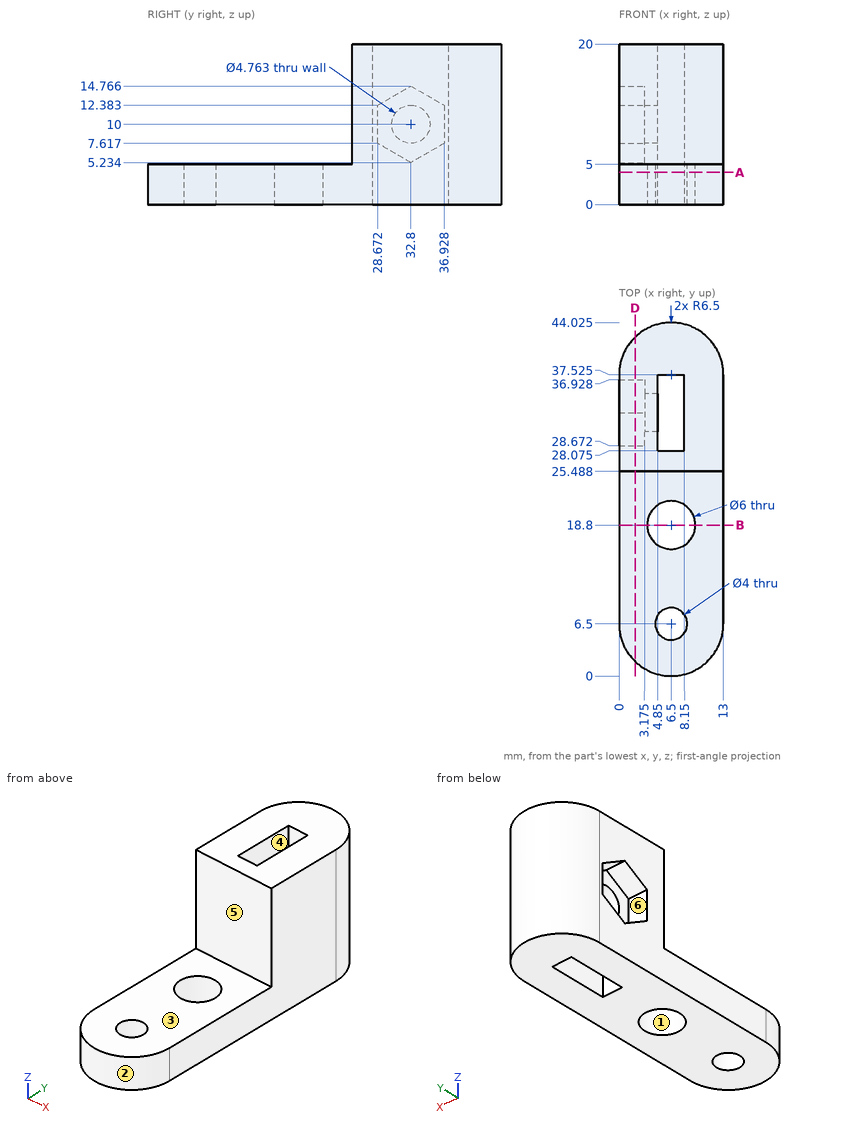
Geometry: see drawing. Coordinates: mm, zero at the bounding-box minimum. A direction names the side the tool comes from. Round coordinates to 2 decimals unless told otherwise and drop trailing zeros. Loops run counter-clockwise (first coordinate to the right, second up) from the corner with the lowest first, then second, coordinate; pieces in that order, holes last. Notation, with made-up numbers: (25.25, 41) - (73.25, 41) arc R17 cw to (73.25, 45) - close; hole circle Ø11 at (59.25, 14.25). An arc over 180 degrees is marked (long way). Write item = value, one per line. Start each with the question number.
(1) Pull-direction query (X, two-part tool) for the marked faces 1, 2 and 3; classes: +X half, -X half, draft (parallel to the pull), parting line (faces both ways), or undercut.
(2) Set-up query: the marked faces 4, 5 and 6. Return all of +Z, -Z, +X, -X, +Y, -Y with unobstructed straight access to the full face (end or side cutting, diameter ignored); none if empty.
(3) Section query A-A, the plane z = 4. State how many separate pieces and enclosed holes the cut face has, plus the area to 3 significant figures.
(4) Pin query (flat end, axial travel): pin 1 (3 mm diameter, centred on y = 30.5, z = 8.5, fed in from -X) (1 decimal); pin 2 (5 mm diameter, centred on x = 3, z = 12, fed in from -Y); pin 3 (1.6 mm diameter, centred on x = 1, z = 11, fed in from +Y) (1 decimal); pin 4 (5 mm diameter, centred on x = 6.5, y = 18.8, fed in from -Z). Return the tip coordinate at first contact, or that it passes through.
(5) Section query D-D, the plane x = 2. Output: boundary loops of the cut face in (y, z) (1 decimal), plus the area to 3 significant figures.
(6) Section query B-B, the plane y = 18.8. Output: boundary loops of the cut face in (x, z).
(7) Ray query, line 1 along Y through (x, z) = (6.5, 1.4) (1 decimal); line 2 along X through (y, z) = (33.5, 3.25); line 3 along Z through (x, y) = (12, 17). Return the intervals inside material, ascending. Write a range as from..to.
Conclusion:
q1.face_1 = undercut
q1.face_2 = parting line
q1.face_3 = draft
q2.face_4 = +Z, -Z
q2.face_5 = +Z, +X, -X, -Y
q2.face_6 = -X
q3.separate_pieces = 1
q3.enclosed_holes = 3
q3.area = 464 mm2
q4.pin_1 = 3.2
q4.pin_2 = 25.49
q4.pin_3 = 42
q4.pin_4 = through
q5.outline = (1.8, 0) - (42.2, 0) - (42.2, 20) - (25.5, 20) - (25.5, 5) - (1.8, 5) - close; hole (28.7, 7.6) - (32.8, 5.2) - (36.9, 7.6) - (36.9, 12.4) - (32.8, 14.8) - (28.7, 12.4) - close
q5.area = 394 mm2
q6.outline = (0, 0) - (3.5, 0) - (3.5, 5) - (0, 5) - close; (9.5, 0) - (13, 0) - (13, 5) - (9.5, 5) - close
q7.line_1 = 0..4.5, 8.5..15.8, 21.8..28.1, 37.5..44
q7.line_2 = 0..4.85, 8.15..13
q7.line_3 = 0..5
